Read the model definition and answer for the solid it produces. Units are mm, in the model's axes. A direction names the side the tool comes from. Round coordinates to 2 decimals unless told otherwise and drop trailing zeros. Order: outer loops, then holes, each group sorted by start corner. A loop starts at its lowest first (then second) coordinate and runs counter-clockwise, first axis right, second up. Notation, with made-up numbers: (55.25, 9) -> (76.25, 9) arc R16 ccw to (76.25, 39) -> close; hole circle Ø11 at (21, -34.75). An arc over 180 degrees is marked (long way). Answer as a JSON object with one key per item and string values. Group by question number.
Item 1: Section A-A, the plane y = 25.6 is taken. Write down the section's boundary in (x, z), plus the area to 3 significant figures.
Item 2: Section B-B, the plane x = -62.5 is taken. Write down the section's boundary in (y, z), plus the area to 3 significant figures.
Item 3: Consider probe 1 along Y at (x, z) = (-62.5, -0.95); probe 2 along X at (y, z) = (-14, -1.5); probe 3 along X at (y, z) = (-0.5, -1.3). Determine where each line is inside the solid, lowest interval first. Write a range as from..to.
Item 4: Given P1, Ø2.5, axis at x = 62.5, y = 25.6, coming from the +Z side; P2, Ø1.5, axis at y = -8.5, z = 2, coming from the -X side; P3, Ø3.5, axis at y = -2, z = 2, coming from the +X side; P4, Ø3.5, axis at x = 6, z = 2, coming from the -Y side, each flat-ended and moving along its own axis, determine where each tip first touches the part or whether it passes through.
Item 5: Section D-D, the plane y = -6 is taken. Write down the section's boundary in (x, z), plus the area to 3 significant figures.
Item 6: The mould has two halves that part along Y. Classify faces 6 (the flat face through (60.4, -23.3, 1.5)), 7 (the flat face through (6.52, 0, 0)), 8 (the flat face through (0, -29, 0)): pulls with the +Y half, pulls with the -Y half, needs draft (parallel to the pull), parting line crosses it, or undercut.
Item 7: Section C-C, the plane z = 2.1 is taken. Write down the section's boundary in (x, y), plus the area to 3 significant figures.
Item 8: For faces 1 (the flat face through (-65.3, 0, 1)), 2 (the flat face through (-60.2, -23.5, 1.5)), 3 (the flat face through (-11.48, 0, 0)), 4 (the flat face through (-1, -28.4, 1)), 5 (the flat face through (14, 0, 3)), determine the directions among +Z, -Z, +X, -X, +Y, -Y from which every point of the face is accessible in a straight line to the end or side of a thin tool.
from build123d import *

# Parameters (mm, degrees)
SKETCH2_W           = 140
SKETCH2_H           = 66.2
BOSS_EXTRUDE1_DEPTH = 3
SKETCH3_W           = 130.6
SKETCH3_H           = 56.8
BOSS_EXTRUDE2_DEPTH = 3
CUT_EXTRUDE1_DEPTH  = 7
SKETCH5_R           = 1.5
CUT_EXTRUDE2_DEPTH  = 7
CUT_EXTRUDE3_DEPTH  = 3


with BuildPart() as part:
    # Sketch2 → Boss-Extrude1 (new body)
    with BuildSketch(Plane.XY):
        Rectangle(SKETCH2_W, SKETCH2_H)
    extrude(amount=-BOSS_EXTRUDE1_DEPTH)

    # Sketch3 → Boss-Extrude2 (add)
    with BuildSketch(Plane.XY):
        Rectangle(SKETCH3_W, SKETCH3_H)
    extrude(amount=BOSS_EXTRUDE2_DEPTH)

    # Sketch4 → Cut-Extrude1 (cut, through all)
    with BuildSketch(Plane(origin=(0, 0, -3), x_dir=(-1, 0, 0), z_dir=(0, 0, -1))):
        with BuildLine():
            ThreePointArc((-15.519758089, 12.871012345), (-18.86120177, 6.939991617), (-20.019758089, 0.231787685))
            ThreePointArc((-20.019758089, 0.231787685), (-18.86120177, -6.476416248), (-15.519758089, -12.407436975))
            Line((-15.519758089, -12.407436975), (-15.519758089, 12.871012345))
        make_face()
        with BuildLine():
            ThreePointArc((-6.519758089, 19.146068004), (-8.839316816, 18.182146563), (-11.019758089, 16.935080773))
            Line((-11.019758089, 16.935080773), (-11.019758089, -16.471505404))
            ThreePointArc((-11.019758089, -16.471505404), (-8.839316816, -17.718571194), (-6.519758089, -18.682492635))
            Line((-6.519758089, -18.682492635), (-6.519758089, 19.146068004))
        make_face()
        with BuildLine():
            ThreePointArc((2.480241911, 20.074922518), (1.232700165, 20.192532869), (-0.019758083, 20.231787685))
            ThreePointArc((-0.019758083, 20.231787685), (-1.021013587, 20.206709147), (-2.019758089, 20.131536427))
            Line((-2.019758089, 20.131536427), (-2.019758089, -19.667961057))
            ThreePointArc((-2.019758089, -19.667961057), (-1.02101359, -19.743133777), (-0.019758089, -19.768212315))
            ThreePointArc((-0.019758089, -19.768212315), (1.232700162, -19.7289575), (2.480241911, -19.611347148))
            Line((2.480241911, -19.611347148), (2.480241911, 20.074922518))
        make_face()
        with BuildLine():
            ThreePointArc((11.480241911, 16.594855857), (9.305959472, 17.924469561), (6.980241911, 18.96678168))
            Line((6.980241911, 18.96678168), (6.980241911, -18.50320631))
            ThreePointArc((6.980241911, -18.50320631), (9.305959472, -17.460894191), (11.480241911, -16.131280487))
            Line((11.480241911, -16.131280487), (11.480241911, 16.594855857))
        make_face()
        with BuildLine():
            ThreePointArc((19.980241911, 0.231787685), (18.953907872, 6.556343005), (15.980241911, 12.231787685))
            Line((15.980241911, 12.231787685), (15.980241911, -11.768212315))
            ThreePointArc((15.980241911, -11.768212315), (18.953907872, -6.092767635), (19.980241911, 0.231787685))
        make_face()
    extrude(amount=-CUT_EXTRUDE1_DEPTH, mode=Mode.SUBTRACT)

    # Sketch5 → Cut-Extrude2 (cut, through all)
    with BuildSketch(Plane(origin=(0, 0, -3), x_dir=(-1, 0, 0), z_dir=(0, 0, -1))):
        with Locations((-62.5, 25.6)):
            Circle(SKETCH5_R)
        with Locations((62.5, 25.6)):
            Circle(SKETCH5_R)
        with Locations((62.5, -25.6)):
            Circle(SKETCH5_R)
        with Locations((-62.5, -25.6)):
            Circle(SKETCH5_R)
    extrude(amount=-CUT_EXTRUDE2_DEPTH, mode=Mode.SUBTRACT)

    # Sketch6 → Cut-Extrude3 (cut)
    with BuildSketch(Plane.XY.offset(3)):
        Polygon((65.3, 28.4), (55.3, 28.4), (65.3, 18.4), align=None)
        Polygon((65.3, -28.4), (65.3, -18.4), (55.3, -28.4), align=None)
        Polygon((-65.3, -28.4), (-55.3, -28.4), (-65.3, -18.4), align=None)
        Polygon((-65.3, 28.4), (-65.3, 18.4), (-55.3, 28.4), align=None)
    extrude(amount=-CUT_EXTRUDE3_DEPTH, mode=Mode.SUBTRACT)


solid = part.part
Values found:
{
 "1": {"outline": "(-70, -3) -> (-64, -3) -> (-64, 0) -> (-70, 0) -> close; (-61, -3) -> (61, -3) -> (61, 0) -> (58.1, 0) -> (58.1, 3) -> (-58.1, 3) -> (-58.1, 0) -> (-61, 0) -> close; (64, -3) -> (70, -3) -> (70, 0) -> (64, 0) -> close", "area": "751 mm2"},
 "2": {"outline": "(-33.1, -3) -> (-27.1, -3) -> (-27.1, 0) -> (-33.1, 0) -> close; (-24.1, -3) -> (24.1, -3) -> (24.1, 0) -> (21.2, 0) -> (21.2, 3) -> (-21.2, 3) -> (-21.2, 0) -> (-24.1, 0) -> close; (27.1, -3) -> (33.1, -3) -> (33.1, 0) -> (27.1, 0) -> close", "area": "308 mm2"},
 "3": {"probe 1": "-33.1..-27.1, -24.1..24.1, 27.1..33.1", "probe 2": "-70..-11.48, -6.98..-2.48, 2.02..6.52, 11.02..70", "probe 3": "-70..-19.97, -15.98..-11.48, -6.98..-2.48, 2.02..6.52, 11.02..15.52, 20.01..70"},
 "4": {"P1": "through", "P2": "x = -65.3", "P3": "x = 65.3", "P4": "y = -28.4"},
 "5": {"outline": "(-70, -3) -> (-18.98, -3) -> (-18.98, 3) -> (-65.3, 3) -> (-65.3, 0) -> (-70, 0) -> close; (-15.98, -3) -> (-11.48, -3) -> (-11.48, 3) -> (-15.98, 3) -> close; (-6.98, -3) -> (-2.48, -3) -> (-2.48, 3) -> (-6.98, 3) -> close; (2.02, -3) -> (6.52, -3) -> (6.52, 3) -> (2.02, 3) -> close; (11.02, -3) -> (15.52, -3) -> (15.52, 3) -> (11.02, 3) -> close; (19.02, -3) -> (70, -3) -> (70, 0) -> (65.3, 0) -> (65.3, 3) -> (19.02, 3) -> close", "area": "692 mm2"},
 "6": {"face 6": "pulls with the -Y half", "face 7": "undercut", "face 8": "needs draft"},
 "7": {"outline": "(-65.3, -18.4) -> (-55.3, -28.4) -> (55.3, -28.4) -> (65.3, -18.4) -> (65.3, 18.4) -> (55.3, 28.4) -> (-55.3, 28.4) -> (-65.3, 18.4) -> close; hole (-15.98, -11.77) -> (-15.98, 12.23) arc R20 ccw to start; hole (-11.48, -16.13) arc R20 ccw to (-6.98, -18.5) -> (-6.98, 18.97) arc R20 ccw to (-11.48, 16.59) -> close; hole (-2.48, -19.61) arc R20 ccw to (2.02, -19.67) -> (2.02, 20.13) arc R20 ccw to (-2.48, 20.07) -> close; hole (6.52, -18.68) arc R20 ccw to (11.02, -16.47) -> (11.02, 16.94) arc R20 ccw to (6.52, 19.15) -> close; hole (15.52, -12.41) arc R20 ccw to (15.52, 12.87) -> close", "area": "6,570 mm2"},
 "8": {"face 1": "+Z, -X, +Y, -Y", "face 2": "+Z, -X, -Y", "face 3": "+Z, -Z", "face 4": "+Z, +X, -X, -Y", "face 5": "+Z, +X, -X, +Y, -Y"}
}
